Source: CAD feature listing. Evaluate the final solid. Frame: model axes, mm. A direction names the side the tool comes from. Round coordinates to 2 decimals unless told otherwise and drop trailing zeros. Write each loop counter-clockwise with the first axis right and the second up, starting at its lowest first coordinate (ties: lowest second). Pieces come first, ordered by that corner, then holes. Notation, with made-up numbers: M 66.25,-10.5 L 125.25,-10.5 A35 ccw 125.25,26.5 Z; hole C 51.25,3.5 d8. An arc over 180 degrees is marked long. Put each result on its own line as item: value. Start each with the question number.
```python
from build123d import *

# Parameters (mm, degrees)
SKETCH_W               = 47.7
SKETCH_H               = 23.7
PAD_DEPTH              = 14.4
SKETCH001_W            = 44.1
SKETCH001_H            = 20.1
POCKET_DEPTH           = 12.6
SKETCH002_R            = 3.6
PAD001_DEPTH           = 2.7
LINEARPATTERN_COUNT    = 4
LINEARPATTERN_PITCH    = 12
SKETCH003_R            = 4.89
SKETCH003_R_2          = 3.6
PAD002_DEPTH           = 12.6
LINEARPATTERN001_COUNT = 3
LINEARPATTERN001_PITCH = 12


with BuildPart() as part:
    # Sketch → Pad (new body)
    with BuildSketch(Plane.XY):
        with Locations((23.85, 11.85)):
            Rectangle(SKETCH_W, SKETCH_H)
    extrude(amount=PAD_DEPTH)

    # Sketch001 (on Face5 of Pad) → Pocket (cut)
    with BuildSketch(Plane(origin=(0, 0, 0), x_dir=(1, 0, 0), z_dir=(0, 0, -1))):
        with Locations((23.85, -11.85)):
            Rectangle(SKETCH001_W, SKETCH001_H)
    extrude(amount=-POCKET_DEPTH, mode=Mode.SUBTRACT)

    # Sketch002 (on Face5 of Pocket) → Pad001 (join)
    with BuildSketch(Plane.XY.offset(14.4)):
        with Locations((6, 17.7)):
            Circle(SKETCH002_R)
        with Locations((6, 6)):
            Circle(SKETCH002_R)
    pad001 = extrude(amount=PAD001_DEPTH)

    # LinearPattern: Pad001 ×4
    with Locations(*[(i * LINEARPATTERN_PITCH, 0, 0) for i in range(1, LINEARPATTERN_COUNT)]):
        add(pad001)

    # Sketch003 (on Face19 of LinearPattern) → Pad002 (join)
    with BuildSketch(Plane(origin=(0, 0, 12.6), x_dir=(1, 0, 0), z_dir=(0, 0, -1))):
        with Locations((12, -12)):
            Circle(SKETCH003_R)
        with Locations((12, -12)):
            Circle(SKETCH003_R_2, mode=Mode.SUBTRACT)
    pad002 = extrude(amount=PAD002_DEPTH)

    # LinearPattern001: Pad002 ×3
    with Locations(*[(i * LINEARPATTERN001_PITCH, 0, 0) for i in range(1, LINEARPATTERN001_COUNT)]):
        add(pad002)


solid = part.part
```
(1) Ray query, line 1 along Y through (x, z) = (12, 6.25); line 2 along X through (y, z) = (6.25, 8); line 3 along Y through (x, z) = (20, 7.75). Return the intervals inside material, ascending.
(2) Contact query for a flat-ended pin moving along its axis: P1, Ø4.5, axis at x = 36, y = 12, coming from the -Z side. Output: stop coordinate, or through.
(3) Section query C-C (x = 24). Return loops of the section in (y, z).
(4) Section query B-B (z = 15.75). Return loops of the section in (x, y).
(5) Section query A-A (z = 5). Return loops of the section in (x, y).
(6) Access query for faces 5 (the flat face through (30, 6, 17.1)), 6 (the cylindrical face through (17.22, 14.186, 15.731)), 7 (the flat face through (18.6, 11.7, 12.6)). Directions: +Z, -Z, +X, -X, +Y, -Y. A direction counts if a zero-diameter tool reaches every point of the face in a straight line with its end or side. Return the directions, or none.
(7) Pull-direction query (X, two-part tool) for faces 1 (the cylindrical face through (20.396, 8.695, 6.388)), 2 (the flat face through (0, 12, 7)), 3 (the flat face through (24, 0, 7)), 4 (the cylindrical face through (7.935, 9.036, 15.731)); classes: +X half, -X half, draft (parallel to the pull), parting line (faces both ways), or undercut.
Entries:
1. line 1: 0 to 1.8, 7.11 to 8.4, 15.6 to 16.89, 21.9 to 23.7
1. line 2: 0 to 1.8, 45.9 to 47.7
1. line 3: 0 to 1.8, 9.19 to 14.81, 21.9 to 23.7
2. P1: z = 12.6
3. outline: M 0,0 L 1.8,0 L 1.8,12.6 L 7.11,12.6 L 7.11,0 L 8.4,0 L 8.4,12.6 L 15.6,12.6 L 15.6,0 L 16.89,0 L 16.89,12.6 L 21.9,12.6 L 21.9,0 L 23.7,0 L 23.7,14.4 L 0,14.4 Z
4. outline: C 6,6 d7.2; C 6,17.7 d7.2; C 18,6 d7.2; C 18,17.7 d7.2; C 30,6 d7.2; C 30,17.7 d7.2; C 42,6 d7.2; C 42,17.7 d7.2
5. outline: M 0,0 L 47.7,0 L 47.7,23.7 L 0,23.7 Z; C 12,12 d9.78; C 24,12 d9.78; C 36,12 d9.78; hole M 1.8,1.8 L 45.9,1.8 L 45.9,21.9 L 1.8,21.9 Z; hole C 12,12 d7.2; hole C 24,12 d7.2; hole C 36,12 d7.2
6. face 5: +Z, +X, -X, +Y, -Y
6. face 6: +Z
6. face 7: -Z
7. face 1: undercut
7. face 2: -X half
7. face 3: draft
7. face 4: undercut
